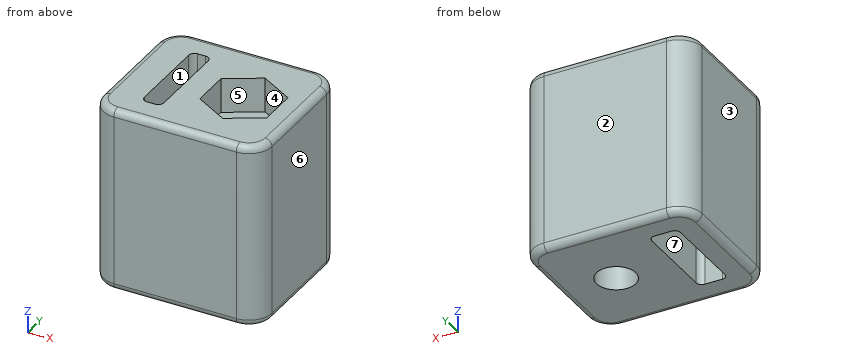
```python
from build123d import *

# Parameters (mm, degrees)
SKETCH1_R           = 1.7
BOSS_EXTRUDE1_DEPTH = 16
CUT_EXTRUDE1_DEPTH  = 3
CUT_EXTRUDE2_DEPTH  = 8
FILLET1_R           = 0.6


with BuildPart() as part:
    # Sketch1 → Boss-Extrude1 (new body)
    with BuildSketch(Plane.XY):
        with BuildLine():
            Line((2, 0), (12.6, 0))
            ThreePointArc((12.6, 0), (14.014213562, 0.585786438), (14.6, 2))
            Line((14.6, 2), (14.6, 10.6))
            ThreePointArc((14.6, 10.6), (14.014213562, 12.014213562), (12.6, 12.6))
            Line((12.6, 12.6), (2, 12.6))
            ThreePointArc((2, 12.6), (0.585786438, 12.014213562), (0, 10.6))
            Line((0, 10.6), (0, 2))
            ThreePointArc((0, 2), (0.585786438, 0.585786438), (2, 0))
        make_face()
        with Locations((9.8, 6.3)):
            Circle(SKETCH1_R, mode=Mode.SUBTRACT)
        with BuildLine():
            Line((3.1, 9.8), (3.1, 2.8))
            ThreePointArc((3.1, 2.8), (3.246446609, 2.446446609), (3.6, 2.3))
            Line((3.6, 2.3), (4.3, 2.3))
            ThreePointArc((4.3, 2.3), (4.653553391, 2.446446609), (4.8, 2.8))
            Line((4.8, 2.8), (4.8, 9.8))
            ThreePointArc((4.8, 9.8), (4.653553391, 10.153553391), (4.3, 10.3))
            Line((4.3, 10.3), (3.6, 10.3))
            ThreePointArc((3.6, 10.3), (3.246446609, 10.153553391), (3.1, 9.8))
        make_face(mode=Mode.SUBTRACT)
    extrude(amount=BOSS_EXTRUDE1_DEPTH)

    # Sketch2 → Cut-Extrude1 (cut)
    with BuildSketch(Plane.XY.offset(16)):
        Polygon((9.8, 9.648631561), (6.9, 7.974315781), (6.9, 4.625684219), (9.8, 2.951368439), (12.7, 4.625684219), (12.7, 7.974315781), align=None)
    extrude(amount=-CUT_EXTRUDE1_DEPTH, mode=Mode.SUBTRACT)

    # Sketch3 → Cut-Extrude2 (cut)
    with BuildSketch(Plane(origin=(0, 0, 0), x_dir=(-1, 0, 0), z_dir=(0, 0, -1))):
        with BuildLine():
            Line((-4.8, 9.8), (-4.8, 2.8))
            ThreePointArc((-4.8, 2.8), (-4.653553391, 2.446446609), (-4.3, 2.3))
            Line((-4.3, 2.3), (-2.8, 2.3))
            ThreePointArc((-2.8, 2.3), (-2.446446609, 2.446446609), (-2.3, 2.8))
            Line((-2.3, 2.8), (-2.3, 9.8))
            ThreePointArc((-2.3, 9.8), (-2.446446609, 10.153553391), (-2.8, 10.3))
            Line((-2.8, 10.3), (-4.3, 10.3))
            ThreePointArc((-4.3, 10.3), (-4.653553391, 10.153553391), (-4.8, 9.8))
        make_face()
    extrude(amount=-CUT_EXTRUDE2_DEPTH, mode=Mode.SUBTRACT)

    # Fillet1
    fillet1_edges = [part.edges().sort_by_distance(p)[0] for p in [
        (0, 6.3, 0),
        (0.585786438, 12.014213562, 0),
        (7.3, 12.6, 0),
        (14.014213562, 12.014213562, 0),
        (0.585786438, 12.014213562, 16),
        (0, 6.3, 16),
        (0.585786438, 0.585786438, 16),
        (7.3, 0, 16),
        (14.014213562, 0.585786438, 16),
        (14.6, 6.3, 16),
        (14.014213562, 12.014213562, 16),
        (14.6, 6.3, 0),
        (7.3, 12.6, 16),
        (14.014213562, 0.585786438, 0),
        (7.3, 0, 0),
        (0.585786438, 0.585786438, 0),
    ]]
    fillet(fillet1_edges, radius=FILLET1_R)


solid = part.part
```
Can you work these out from the model? Positions are in its coordinate system, mm. Face numbers are marked on the shaded views. A direction names the side the tool comes from. Coordinates: 2 decimals unless noted, no trailing zeros. Loops run counter-clockwise (first coordinate to the right, second up) from the corner with the lowest first, then second, coordinate; pieces in that order, holes last. Notation, with made-up numbers: (56, -24) -> (97, -24) arc R22 ccw to (97, -1) -> close; hole circle Ø6 at (71.5, 52.5). An arc over 180 degrees is marked (long way). Put each result on its own line as item: value. Start each with the question number.
Q1. Thinking about a two-plate mould opening in X: for the marked faces 1, 2, 3 and 4, which applies, pulls with the +X half, pulls with the -X half, needs draft (parallel to the pull), parting line crosses it, or undercut?
Q2. I want a section at C-C (x = 9.5). Write out the boundary of the cut face in (y, z), plus the area to 3 significant figures.
Q3. I want a section at D-D (y = 8.5). Write out the boundary of the cut face in (x, z).
Q4. I want a section at B-B (y = 6.3). Write out the boundary of the cut face in (x, z), plus the area to 3 significant figures.
Q5. For the marked faces 5, 6 and 7, which set-ups out of +Z, -Z, +X, -X, +Y, -Y let a thin tool reach every point of the face, with its end or its side?
Q6. I'm going to push a flat-ended pin straight in: P1, Ø1.7, axis at x = 8.5, y = 7.5, coming from the +Z side. Where does the tip first touch, or does it pass through?
Q7. I want a section at A-A (z = 6). Write out the boundary of the cut face in (x, y).
Q8. If I drill on line 1 (X direction, y = 7.5, z = 13.75); line 2 (X direction, y = 6.3, z = 10); line 3 (Y direction, x = 9.8, z = 7), over which ranges is the centre line in solid material (lowest first)? Write a range as [from, to].
Taken from the geometry:
1. face 1: undercut
1. face 2: needs draft
1. face 3: pulls with the -X half
1. face 4: undercut
2. outline: (0, 0.6) arc R0.6 ccw to (0.6, 0) -> (4.63, 0) -> (4.63, 13) -> (3.12, 13) -> (3.12, 16) -> (0.6, 16) arc R0.6 ccw to (0, 15.4) -> close; (7.97, 0) -> (12, 0) arc R0.6 ccw to (12.6, 0.6) -> (12.6, 15.4) arc R0.6 ccw to (12, 16) -> (9.48, 16) -> (9.48, 13) -> (7.97, 13) -> close
2. area: 139 mm2
3. outline: (0, 0.6) arc R0.6 ccw to (0.6, 0) -> (2.3, 0) -> (2.3, 8) -> (3.1, 8) -> (3.1, 16) -> (0.6, 16) arc R0.6 ccw to (0, 15.4) -> close; (4.8, 0) -> (14, 0) arc R0.6 ccw to (14.6, 0.6) -> (14.6, 15.4) arc R0.6 ccw to (14, 16) -> (11.79, 16) -> (11.79, 13) -> (7.81, 13) -> (7.81, 16) -> (4.8, 16) -> close
4. outline: (0, 0.6) arc R0.6 ccw to (0.6, 0) -> (2.3, 0) -> (2.3, 8) -> (3.1, 8) -> (3.1, 16) -> (0.6, 16) arc R0.6 ccw to (0, 15.4) -> close; (4.8, 0) -> (8.1, 0) -> (8.1, 13) -> (6.9, 13) -> (6.9, 16) -> (4.8, 16) -> close; (11.5, 0) -> (14, 0) arc R0.6 ccw to (14.6, 0.6) -> (14.6, 15.4) arc R0.6 ccw to (14, 16) -> (12.7, 16) -> (12.7, 13) -> (11.5, 13) -> close
4. area: 138 mm2
5. face 5: +Z
5. face 6: +Z, -Z, +X, +Y, -Y
5. face 7: +Z, -Z
6. P1: stops at z = 13
7. outline: (0, 2) arc R2 ccw to (2, 0) -> (12.6, 0) arc R2 ccw to (14.6, 2) -> (14.6, 10.6) arc R2 ccw to (12.6, 12.6) -> (2, 12.6) arc R2 ccw to (0, 10.6) -> close; hole (2.3, 2.8) arc R0.5 ccw to (2.8, 2.3) -> (4.3, 2.3) arc R0.5 ccw to (4.8, 2.8) -> (4.8, 9.8) arc R0.5 ccw to (4.3, 10.3) -> (2.8, 10.3) arc R0.5 ccw to (2.3, 9.8) -> close; hole circle Ø3.4 at (9.8, 6.3)
8. line 1: x = [0, 3.1], [4.8, 6.9], [12.7, 14.6]
8. line 2: x = [0, 3.1], [4.8, 8.1], [11.5, 14.6]
8. line 3: y = [0, 4.6], [8, 12.6]
